```python
from build123d import *

# Parameters (mm, degrees)
BOSS_EXTRUDE1_DEPTH = 3
SKETCH3_W           = 27
SKETCH3_H           = 6.5
SKETCH3_R           = 1.6
BOSS_EXTRUDE2_DEPTH = 3


with BuildPart() as part:
    # Sketch1 → Boss-Extrude1 (new body)
    with BuildSketch(Plane.XY):
        with BuildLine():
            Line((2.5, -87.48740775), (2.5, -12.247448714))
            ThreePointArc((2.5, -12.247448714), (12.259414932, -2.440644491), (7, 10.356157589))
            Line((7, 10.356157589), (-7, 10.356157589))
            ThreePointArc((-7, 10.356157589), (-12.259414932, -2.440644491), (-2.5, -12.247448714))
            Line((-2.5, -12.247448714), (-2.5, -87.48740775))
            Line((-2.5, -87.48740775), (2.5, -87.48740775))
        make_face()
        with BuildLine():
            ThreePointArc((7, -7.487489566), (10.25, 0), (7, 7.487489566))
            Line((7, 7.487489566), (-7, 7.487489566))
            ThreePointArc((-7, 7.487489566), (-10.25, 0), (-7, -7.487489566))
            Line((-7, -7.487489566), (7, -7.487489566))
        make_face(mode=Mode.SUBTRACT)
    extrude(amount=BOSS_EXTRUDE1_DEPTH)

    # Sketch3 → Boss-Extrude2 (add)
    with BuildSketch(Plane.XY):
        with Locations((0, -30.497448714)):
            Rectangle(SKETCH3_W, SKETCH3_H)
        with Locations((-10.3, -30.497448714)):
            Circle(SKETCH3_R, mode=Mode.SUBTRACT)
        with Locations(Location((10.3, -30.497448714, 0), (0, 0, 180))):
            Circle(SKETCH3_R, mode=Mode.SUBTRACT)
    extrude(amount=BOSS_EXTRUDE2_DEPTH)


solid = part.part
```
Part model, mm, in its own coordinate system. A direction names the side the tool comes from. Coordinates: 2 decimals unless noted, no trailing zeros. Write each loop counter-clockwise with the first axis right and the second up, starting at its lowest first coordinate (ties: lowest second). Pieces come first, ordered by that corner, then holes.
Item 1: Which spindle directions (+Z, -Z, +X, -X, +Y, -Y) get a long thin tool onto all of the face, cutting with end or side? Do faces 5 (the face through (0, 7.487, 1)), 6 (the face through (-2.5, -60, 1)), 7 (the face through (2.5, -20, 1)), 8 (the face through (2.5, -61, 1)), 9 (the face through (-2.5, -20, 1)). Say none if no direction does.
Item 2: Mould opens along X. For faces 1 (the face through (-1, -35, 3)), 2 (the face through (-9.562, -31.917, 1.479)), 3 (the face through (13.5, -31, 1)), 4 (the face through (-13.5, -31, 1)) say: released by +X, released by -X, zero draft, split by the parting line, or undercut.
Item 3: Probe line 1 (Y direction, x = -10.3, z = 1.5); line 2 (Y direction, x = 9, z = 0.8); line 3 (Y direction, x = 5.25, z = 2.9). List the from-to ranges inside material, lowest first.
Item 4: Pin check, flat tips, straight feed: pin 1 (1.5 mm diameter, centred on x = -6, z = 1.5, fed in from -Y); pin 2 (1.5 mm diameter, centred on y = -22, z = 1.5, fed in from -X); pin 3 (1.5 mm diameter, centred on y = -48, z = 2, fed in from +X); pin 4 (2 mm diameter, centred on x = -4, y = -24, fed in from -Z). Stop position of each tip, or through.
Item 5: Slice it at C-C (z = 0.7). Write the cut outline in (x, y).
Item 6: Slice it at B-B (x = 5). Write the cut outline in (y, z), and give its area (3 significant figures).
Item 7: Slice it at D-D (y = -56). Write the cut outline in (x, z).
Item 8: Slice it at A-A (y = 0). Write the cut outline in (x, z).
Results found:
1. face 5: +Z, -Z
1. face 6: +Z, -Z, -X, -Y
1. face 7: +Z, -Z, +X
1. face 8: +Z, -Z, +X, -Y
1. face 9: +Z, -Z, -X
2. face 1: zero draft
2. face 2: undercut
2. face 3: released by +X
2. face 4: released by -X
3. line 1: y = -33.75 to -32.1, -28.9 to -27.25, -7.08 to 7.08
3. line 2: y = -33.75 to -31.43, -29.56 to -27.25, -8.67 to -4.91, 4.91 to 8.67
3. line 3: y = -33.75 to -27.25, -11.34 to -7.49, 7.49 to 10.36
4. pin 1: stops at y = -33.75
4. pin 2: stops at x = -2.5
4. pin 3: stops at x = 2.5
4. pin 4: passes through
5. outline: (-13.5, -33.75) - (-2.5, -33.75) - (-2.5, -87.49) - (2.5, -87.49) - (2.5, -33.75) - (13.5, -33.75) - (13.5, -27.25) - (2.5, -27.25) - (2.5, -12.25) arc R12.5 ccw to (7, 10.36) - (-7, 10.36) arc R12.5 ccw to (-2.5, -12.25) - (-2.5, -27.25) - (-13.5, -27.25) - close; hole circle Ø3.2 at (-10.3, -30.5); hole (-7, -7.49) - (7, -7.49) arc R10.25 ccw to (7, 7.49) - (-7, 7.49) arc R10.25 ccw to start; hole circle Ø3.2 at (10.3, -30.5)
6. outline: (-33.75, 0) - (-27.25, 0) - (-27.25, 3) - (-33.75, 3) - close; (-11.46, 0) - (-7.49, 0) - (-7.49, 3) - (-11.46, 3) - close; (7.49, 0) - (10.36, 0) - (10.36, 3) - (7.49, 3) - close
6. area: 40.0 mm2
7. outline: (-2.5, 0) - (2.5, 0) - (2.5, 3) - (-2.5, 3) - close
8. outline: (-12.5, 0) - (-10.25, 0) - (-10.25, 3) - (-12.5, 3) - close; (10.25, 0) - (12.5, 0) - (12.5, 3) - (10.25, 3) - close
